Can you work these out from the model? Positions are in its coordinate system, mm. A direction names the side the tool comes from. Round coordinates to 2 decimals unless told otherwise and drop trailing zeros. Loops run counter-clockwise (first coordinate to the right, second up) from the corner with the lowest first, then second, coordinate; pieces in that order, holes last.
from build123d import *

# Parameters (mm, degrees)
F0_W            = 76.2
F0_H            = 50.8
F1_DEPTH        = 25.4
F3_DEPTH        = 25.401
F5_D            = 9.525
F7_DEPTH        = 25.401
F9_DEPTH        = 25.401
F11_DEPTH       = 25.4
F13_D           = 3.175
F15_DEPTH       = 46.99
F17_D           = 4.1656
F17_CBORE_D     = 9.525
F17_CBORE_DEPTH = 3.81


with BuildPart() as f1:
    # F0 (on Front) → F1 (new body)
    with BuildSketch(Plane.XZ):
        Rectangle(F0_W, F0_H)
    extrude(amount=F1_DEPTH)

    # F2 (on face) → F3 (cut, through all)
    with BuildSketch(Plane.XZ.offset(25.4)):
        Polygon((38.1, -25.4), (38.1, 25.4), (24.4881810245, -25.4), align=None)
    extrude(amount=-F3_DEPTH, mode=Mode.SUBTRACT)

    # F5 (through all)
    with Locations(Plane(origin=(29.1977839421, 0, -7.8235226281), x_dir=(0, 1, 0), z_dir=(0.9659258263, 0, -0.2588190451))):
        with Locations((-12.7, 22.0410656184)):
            Hole(F5_D / 2)

    # F6 (on face) → F7 (cut, through all)
    with BuildSketch(Plane(origin=(0, 0, 0), x_dir=(-1, 0, 0), z_dir=(0, 1, 0))):
        Polygon((-24.4881810245, 25.4), (-38.1, 25.4), (-24.4881810245, -25.4), align=None)
    extrude(amount=-F7_DEPTH, mode=Mode.SUBTRACT)

    # F8 (on face) → F9 (cut, through all)
    with BuildSketch(Plane.XZ.offset(25.4)):
        Polygon((24.4881810245, -25.4), (24.4881810245, 25.4), (10.876362049, -25.4), align=None)
    extrude(amount=-F9_DEPTH, mode=Mode.SUBTRACT)

    # F10 (on face) → F11 (join)
    with BuildSketch(Plane.XZ.offset(25.4)):
        Polygon((44.4944761693, 25.4), (24.4881810245, 25.4), (10.876362049, -25.4), (44.4944761693, -25.4), align=None)
    extrude(amount=-F11_DEPTH)

    # F13 (through all)
    with Locations(Plane(origin=(16.4977839421, 0, -4.4205678842), x_dir=(0, -1, 0), z_dir=(-0.9659258263, 0, 0.2588190451))):
        with Locations((12.7, 22.0410656184)):
            Hole(F13_D / 2)

    # F14 (on face) → F15 (cut)
    with BuildSketch(Plane.XY.offset(25.4)):
        with BuildLine():
            ThreePointArc((27.7756870478, -25.4), (23.0131870478, -20.6375), (18.2506870478, -25.4))
            Line((18.2506870478, -25.4), (27.7756870478, -25.4))
        make_face()
    extrude(amount=-F15_DEPTH, mode=Mode.SUBTRACT)

    # F17 (through all)
    with Locations(Plane.XZ.offset(25.4)):
        with Locations((-25.4, -12.7), (-25.4, 12.7), (0, 0)):
            CounterBoreHole(F17_D / 2, F17_CBORE_D / 2, F17_CBORE_DEPTH)


solid = f1.part
(1) If we section it at C-C, the plane z = -16.5: List the corners of the cut face in (x, y) for me (1 decimal).
Worked answers:
outline: (-38.1, -25.4) - (-28.3, -25.4) - (-28.3, -21.6) - (-22.5, -21.6) - (-22.5, -25.4) - (18.3, -25.4) arc R4.8 cw to (27.8, -25.4) - (44.5, -25.4) - (44.5, 0) - (-38.1, 0) - close
(2) If we section it at D-D, the plane x = -25.4: State how many separate pieces and enclosed holes the cut face has, then the cut area to 3 significant figures.
Worked answers:
separate pieces: 3
enclosed holes: 0
area: 1,040 mm2
(3) If we section it at B-B, the plane y = -12: List the corners of the cut face in (x, z) for me (3 decimals).
Worked answers:
outline: (-38.1, -25.4) - (44.494, -25.4) - (44.494, 9.421) - (21.834, 15.493) - (20.983, 12.319) - (-27.835, 25.4) - (-38.1, 25.4) - close; (8.567, 25.4) - (23.422, 21.42) - (22.571, 18.246) - (44.494, 12.371) - (44.494, 25.4) - close; hole circle Ø4.166 at (-25.4, -12.7); hole circle Ø4.166 at (-25.4, 12.7); hole circle Ø4.166 at (0, 0)
(4) If we section it at A-A, the plane z = 0: List the corners of the cut face in (x, y) for me (1 decimal).
Worked answers:
outline: (-38.1, -25.4) - (-4.8, -25.4) - (-4.8, -21.6) - (-2.1, -21.6) - (-2.1, 0) - (-38.1, 0) - close; (2.1, -21.6) - (4.8, -21.6) - (4.8, -25.4) - (18.3, -25.4) arc R4.8 cw to (27.8, -25.4) - (44.5, -25.4) - (44.5, 0) - (2.1, 0) - close
(5) If we mould it in two halves opening along Y, with no side actions, what happens to faces 5 (the cylindrical face through (-3.78, -23.52, -2.9)), 6 (the cylindrical face through (1.462, -11.668, 17.614)), 7 (the flat face through (3, -25.4, -5)), 8 (the flat face through (3, 0, 0))? For each: released by +Y, released by -Y, zero draft, split by the parting line, or undercut.
Worked answers:
face 5: zero draft
face 6: undercut
face 7: released by -Y
face 8: released by +Y
(6) If I drill on line 1 (Z direction, x = -25.4, y = -16.25); line 2 (Z direction, x = 0, y = -24.1); line 3 (X direction, y = -10, z = 0.5), over which ranges is the centre line in solid material (lowest first)?
Worked answers:
line 1: z = -25.4 to -14.78, -10.62 to 10.62, 14.78 to 25.4
line 2: z = -25.4 to -4.76, 4.76 to 25.4
line 3: x = -38.1 to -2.02, 2.02 to 44.49
(7) Will these pins go through, and if not, where does the flat tip stop? P1, Ø5, axis at x = -25.4, z = 12.7, coming from the -Y side; P2, Ø3.5, axis at x = 0, z = 0, coming from the -Y side.
Worked answers:
P1: stops at y = -21.59
P2: passes through
(8) For faces 1 (the flat face through (4, -7, 25.4)), 2 (the cylindrical face through (23.12, -20.64, 2.23)), 3 (the flat face through (-23, -21.59, 12)), 4 (the flat face through (21.67, -12.77, 14.89)), which set-ups out of +Z, -Z, +X, -X, +Y, -Y let a thin tool reach every point of the face, with its end or its side?
Worked answers:
face 1: +Z, +X, -X, +Y, -Y
face 2: +Z, -Y
face 3: -Y
face 4: none
